```python
from build123d import *

# Parameters (mm, degrees)
SKETCH2_R           = 0.25
BOSS_EXTRUDE1_DEPTH = 10
SKETCH3_R           = 0.25
BOSS_EXTRUDE2_DEPTH = 12


with BuildPart() as part:
    # Sketch1 → Revolve1 (revolve)
    with BuildSketch(Plane.XY, mode=Mode.PRIVATE) as revolve1_sk:
        with BuildLine():
            Line((0, 0), (0, 9.7))
            ThreePointArc((0, 9.7), (1.767766953, 8.967766953), (2.5, 7.2))
            Line((2.5, 7.2), (2.5, 1))
            Line((2.5, 1), (2.95, 1))
            Line((2.95, 1), (2.95, 0))
            Line((2.95, 0), (0, 0))
        make_face()
    revolve(revolve1_sk.sketch.rotate(Axis((0, 0, 0), (0, 1, 0)), 90), axis=Axis((0, 0, 0), (0, 1, 0)))

    # Sketch2 → Boss-Extrude1 (add)
    with BuildSketch(Plane.XZ):
        with Locations(Location((1.27, 0, 0), (0, 0, 270))):
            Circle(SKETCH2_R)
    extrude(amount=BOSS_EXTRUDE1_DEPTH)

    # Sketch3 → Boss-Extrude2 (add)
    with BuildSketch(Plane.XZ):
        with Locations(Location((-1.27, 0, 0), (0, 0, 270))):
            Circle(SKETCH3_R)
    extrude(amount=BOSS_EXTRUDE2_DEPTH)


solid = part.part
```
The model under review builds one solid part; all positions refer to its coordinate system, in mm. A direction names the side the tool comes from. Give positions to 0.01 mm unless a question says otherwise; leave off trailing zeros. Write each loop counter-clockwise with the first axis right and the second up, starting at its lowest first coordinate (ties: lowest second). Pieces come first, ordered by that corner, then holes. Notation, with made-up numbers: M 19,75.25 L 47,75.25 A19 cw 47,103.25 Z; hole C 60,88.25 d9. An arc over 180 degrees is marked long. Write each question's results on one line, items separated by ' | '. Start each with the question number.
1. We need section D-D (y = -10.25). Write out the cut boundary in (x, z).
2. Insertion check: pin 1 Ø2 at (x, z) = (1.5, 1.5) entering from -Y; pin 2 Ø2 at (y, z) = (6.5, -1.5) entering from -X; pin 3 Ø1.5 at (y, z) = (2, -2.5) entering from -X. Each pin has a flat end and moves straight along its axis. Give the tip position at first contact, or say it passes through.
3. For probe 1 along Z at (x, y) = (-0.1, 6.75); probe 2 along Y at (x, z) = (-2.25, 0); probe 3 along Z at (x, y) = (-0.95, 4.5), list the stretches that pass through material, from the lowest coordinate up. Write a range as [from, to].
4. We need section A-A (y = -4.75). Write out the cut boundary in (x, z).
5. We need section B-B (z = 0). Write out the cut boundary in (x, y).
6. For faces 1 (the cylindrical face through (-0.1, 4.1, 2.5)), 2 (the cylindrical face through (-0.13, 0.493, 2.947)), list the 3-axis set-ups (+Z, -Z, +X, -X, +Y, -Y) from which the entire face can be reached by the end or side of a thin tool; tool diameter is ignored.
7. We need section C-C (x = 0). Write out the cut boundary in (y, z), and give its area (3 significant figures).
Results found:
1) outline: C -1.27,0 d0.5
2) pin 1: stops at y = 0 | pin 2: stops at x = -2.45 | pin 3: stops at x = -1.79
3) probe 1: z = [-2.5, 2.5] | probe 2: y = [0, 8.29] | probe 3: z = [-2.31, 2.31]
4) outline: C -1.27,0 d0.5; C 1.27,0 d0.5
5) outline: M -2.95,0 L -1.52,0 L -1.52,-12 L -1.02,-12 L -1.02,0 L 1.02,0 L 1.02,-10 L 1.52,-10 L 1.52,0 L 2.95,0 L 2.95,1 L 2.5,1 L 2.5,7.2 A2.5 ccw -2.5,7.2 L -2.5,1 L -2.95,1 Z
6) face 1: +Y | face 2: +Y, -Y
7) outline: M 0,-2.95 L 1,-2.95 L 1,-2.5 L 7.2,-2.5 A2.5 ccw 7.2,2.5 L 1,2.5 L 1,2.95 L 0,2.95 Z | area: 46.7 mm^2
